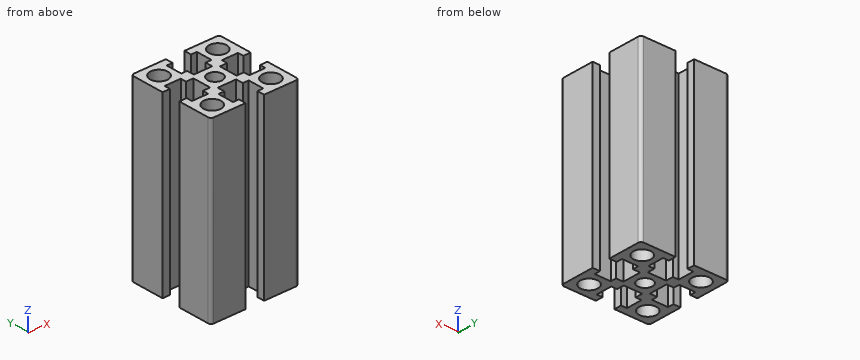
Autodesk Inventor part; units mm, degrees
ref_plane "YZ Plane" through (0, 0, 0) normal (1, 0, 0) x (0, 1, 0)
ref_plane "XZ Plane" through (0, 0, 0) normal (0, 1, 0) x (-1, 0, 0)
ref_plane "XY Plane" through (0, 0, 0) normal (0, 0, 1) x (1, 0, 0)
feature "ソリッド1" [suppressed]
sketch "スケッチ2" plane through (0, 0, 0) normal (0, 0, 1) x (1, 0, 0)
  line L0 (-12.5, 5.15) -> (-7, 5.15)
  line L1 (-7, 5.15) -> (-7, 3.15)
  line L2 (-7, 3.15) -> (-4.5, 3.15)
  line L3 (-4.5, 3.15) -> (-4.5, -3.15)
  line L4 (-4.5, -3.15) -> (-7, -3.15)
  line L5 (-7, -3.15) -> (-7, -5.15)
  line L6 (-7, -5.15) -> (-12.5, -5.15)
  line L7 (-12.5, -5.15) -> (-12.5, -3.15)
  line L8 (-12.5, -3.15) -> (-15, -3.15)
  line L9 (-15, -3.15) -> (-15, -14)
  arc A0 (-15, -14) -> (-14, -15) centre (-14, -14) ccw
  line L10 (-14, -15) -> (-3.15, -15)
  line L11 (-3.15, -15) -> (-3.15, -12.5)
  line L12 (-3.15, -12.5) -> (-5.15, -12.5)
  line L13 (-5.15, -12.5) -> (-5.15, -7)
  line L14 (-5.15, -7) -> (-3.15, -7)
  line L15 (-3.15, -7) -> (-3.15, -4.5)
  line L16 (-3.15, -4.5) -> (3.15, -4.5)
  line L17 (3.15, -4.5) -> (3.15, -7)
  line L18 (3.15, -7) -> (5.15, -7)
  line L19 (5.15, -7) -> (5.15, -12.5)
  line L20 (5.15, -12.5) -> (3.15, -12.5)
  line L21 (3.15, -12.5) -> (3.15, -15)
  line L22 (3.15, -15) -> (14, -15)
  arc A1 (14, -15) -> (15, -14) centre (14, -14) ccw
  line L23 (15, -14) -> (15, -3.15)
  line L24 (15, -3.15) -> (12.5, -3.15)
  line L25 (12.5, -3.15) -> (12.5, -5.15)
  line L26 (12.5, -5.15) -> (7, -5.15)
  line L27 (7, -5.15) -> (7, -3.15)
  line L28 (7, -3.15) -> (4.5, -3.15)
  line L29 (4.5, -3.15) -> (4.5, 3.15)
  line L30 (4.5, 3.15) -> (7, 3.15)
  line L31 (7, 3.15) -> (7, 5.15)
  line L32 (7, 5.15) -> (12.5, 5.15)
  line L33 (12.5, 5.15) -> (12.5, 3.15)
  line L34 (12.5, 3.15) -> (15, 3.15)
  line L35 (15, 3.15) -> (15, 14)
  arc A2 (15, 14) -> (14, 15) centre (14, 14) ccw
  line L36 (14, 15) -> (3.15, 15)
  line L37 (3.15, 15) -> (3.15, 12.5)
  line L38 (3.15, 12.5) -> (5.15, 12.5)
  line L39 (5.15, 12.5) -> (5.15, 7)
  line L40 (5.15, 7) -> (3.15, 7)
  line L41 (3.15, 7) -> (3.15, 4.5)
  line L42 (3.15, 4.5) -> (-3.15, 4.5)
  line L43 (-3.15, 4.5) -> (-3.15, 7)
  line L44 (-3.15, 7) -> (-5.15, 7)
  line L45 (-5.15, 7) -> (-5.15, 12.5)
  line L46 (-5.15, 12.5) -> (-3.15, 12.5)
  line L47 (-3.15, 12.5) -> (-3.15, 15)
  line L48 (-3.15, 15) -> (-14, 15)
  arc A3 (-14, 15) -> (-15, 14) centre (-14, 14) ccw
  line L49 (-15, 14) -> (-15, 3.15)
  line L50 (-15, 3.15) -> (-12.5, 3.15)
  line L51 (-12.5, 3.15) -> (-12.5, 5.15)
  circle A4 centre (10, 10) radius 3
  circle A5 centre (-10, 10) radius 3
  circle A6 centre (-10, -10) radius 3
  circle A7 centre (10, -10) radius 3
  circle A8 centre (0, 0) radius 2.5
extrude "押し出し1" add sketch "スケッチ2" along normal blind 60
equation "\"d1\" = L"
equation "\"L\" = 60"
properties part number "AFS-3030-60"
Geometry: final body of the model. Coordinates: model frame, mm. Give positions to 0.01 mm unless a question says otherwise; leave off trailing zeros. Loops run counter-clockwise (first coordinate to the right, second up) from the corner with the lowest first, then second, coordinate; pieces in that order, holes last. Notation, with made-up numbers: (78.25, 1.25) - (112.25, 1.25) arc R27 cw to (112.25, 25.25) - close; hole circle Ø7 at (-38, -4.5). An arc over 180 degrees is marked (long way). One line per question, with ' | ' between items. Start each with the question number.
(1) Section query B-B on x = 10. Return loops of the section in (y, z), then the cut area to 3 significant figures.
(2) Section query A-A on x = 0. Return loops of the section in (y, z).
(3) Ray query, line 1 (Y direction, x = -4.75, z = 44); line 2 (Y direction, x = -10, z = 38.5); line 3 (X direction, y = -3.75, z = 41). Return the intervals inside material, ascending. Write a range as from..to.
(4) Section query D-D on z = 27.5. Count the separate pieces of the cut face and the enclosed holes in it, then the cut area to 3 significant figures.
(5) Contact query for a flat-ended pin moving along its axis: pin 1 (1.5 mm diameter, centred on y = 1.5, z = 6.5, fed in from +X). Output: stop coordinate, or through.
The answers:
1) outline: (-15, 0) - (-13, 0) - (-13, 60) - (-15, 60) - close; (-7, 0) - (-5.15, 0) - (-5.15, 60) - (-7, 60) - close; (5.15, 0) - (7, 0) - (7, 60) - (5.15, 60) - close; (13, 0) - (15, 0) - (15, 60) - (13, 60) - close | area: 462 mm2
2) outline: (-4.5, 0) - (-2.5, 0) - (-2.5, 60) - (-4.5, 60) - close; (2.5, 0) - (4.5, 0) - (4.5, 60) - (2.5, 60) - close
3) line 1: -15..-12.5, -7..-3.15, 3.15..7, 12.5..15 | line 2: -15..-13, -7..-5.15, 5.15..7, 13..15 | line 3: -15..-12.5, -7..7, 12.5..15
4) separate pieces: 1 | enclosed holes: 5 | area: 414 mm2
5) pin 1: x = 4.5
